Work out the finished part from the listing and answer in its coordinate system (mm). A direction names the side the tool comes from. Round coordinates to 2 decimals unless told otherwise and drop trailing zeros. Write each loop counter-clockwise with the first axis right and the second up, starting at its lowest first coordinate (ties: lowest second). Pieces come first, ordered by that corner, then holes. Notation, with made-up numbers: (-14, -10) - (2, -10) arc R17 cw to (2, -6) - close; hole circle Ø8 at (4.25, 8.5). An arc over 180 degrees is marked (long way). Answer as a JSON object with one key per item and string values.
```python
from build123d import *

# Parameters (mm, degrees)
SKETCH1_R                = 61.7
SEAT_DISC_DEPTH          = 2.8
REAR_STOP_ARC_DEPTH      = 3
SKETCH3_W                = 14
SKETCH3_H                = 23
FRONT_DRAIN_GROOVE_DEPTH = 0.85
SKETCH4_R                = 1
PIN_HOLES_DEPTH          = 1.25


with BuildPart() as part:
    # Sketch1 → Seat_disc (new body)
    with BuildSketch(Plane.XY.offset(72)):
        with Locations((70, 0)):
            Circle(SKETCH1_R)
    extrude(amount=SEAT_DISC_DEPTH)

    # Sketch2 → Rear_stop_arc (add)
    with BuildSketch(Plane.XY.offset(74.8)):
        with BuildLine():
            Line((126.265179381, 15.076209377), (129.597623482, 15.969135083))
            ThreePointArc((129.597623482, 15.969135083), (70, 61.7), (10.402376518, 15.969135083))
            Line((10.402376518, 15.969135083), (13.734820619, 15.076209377))
            ThreePointArc((13.734820619, 15.076209377), (70, 58.25), (126.265179381, 15.076209377))
        make_face()
    extrude(amount=REAR_STOP_ARC_DEPTH)

    # Sketch3 → Front_drain_groove (cut, symmetric)
    with BuildSketch(Plane.XY.offset(74.45)):
        with Locations((70, -51.5)):
            Rectangle(SKETCH3_W, SKETCH3_H)
    extrude(amount=FRONT_DRAIN_GROOVE_DEPTH, both=True, mode=Mode.SUBTRACT)

    # Sketch4 → Pin_holes (cut, symmetric)
    with BuildSketch(Plane.XY.offset(72.75)):
        with Locations((70, 50)):
            Circle(SKETCH4_R)
        with Locations((26.698729811, -25)):
            Circle(SKETCH4_R)
        with Locations((113.301270189, -25)):
            Circle(SKETCH4_R)
    extrude(amount=PIN_HOLES_DEPTH, both=True, mode=Mode.SUBTRACT)


solid = part.part
```
Item 1: Determine the mould class of faces 4 (the flat face through (127.908, 15.516, 76.279)), 5 (the flat face through (70, -51, 73.6)), 6 (the cylindrical face through (61.968, 61.175, 74.215)) for opening direction X: pulls with the +X half, pulls with the -X half, needs draft (parallel to the pull), parting line crosses it, or undercut.
Results found:
{"face 4": "pulls with the +X half", "face 5": "undercut", "face 6": "parting line crosses it"}
Item 2: Each of these flat-tipped pins is pushed along its axis until it touches: P1, Ø2.5, axis at x = 113.3, y = -25, coming from the +Z side; P2, Ø1.3, axis at y = -54.5, z = 74.5, coming from the +X side; P3, Ø0.6, axis at x = 27, y = -25, coming from the -Z side. Where does it stop, or does it pass through?
Results found:
{"P1": "z = 74.8", "P2": "x = 100.12", "P3": "z = 74"}
Item 3: A cutting plane is placed at B-B (x = 23). Write down the section's boundary in (y, z), and give its area (3 significant figures).
Results found:
{"outline": "(-39.97, 72) - (39.97, 72) - (39.97, 77.8) - (34.41, 77.8) - (34.41, 74.8) - (-39.97, 74.8) - close", "area": "241 mm²"}
Item 4: For faces 1 (the cylindrical face through (68.93, 58.24, 76.28)), 2 (the flat face through (70, 59, 77.8)), 3 (the flat face through (12.045, 15.529, 76.279)), determine the directions among +Z, -Z, +X, -X, +Y, -Y from which every point of the face is accessible in a straight line to the end or side of a thin tool.
Results found:
{"face 1": "+Z, -Y", "face 2": "+Z, +X, -X, +Y, -Y", "face 3": "+Z, -X, -Y"}
Item 5: A cutting plane is placed at C-C (y = 31). Write down the section's boundary in (x, z), and give its area (3 significant figures).
Results found:
{"outline": "(16.65, 72) - (123.35, 72) - (123.35, 77.8) - (119.32, 77.8) - (119.32, 74.8) - (20.68, 74.8) - (20.68, 77.8) - (16.65, 77.8) - close", "area": "323 mm²"}
Item 6: A cutting plane is placed at A-A (y = 0). Write down the section's boundary in (x, z).
Results found:
{"outline": "(8.3, 72) - (131.7, 72) - (131.7, 74.8) - (8.3, 74.8) - close"}
Item 7: Consider line 1 along Y through (x, z) = (70, 72.25); line 2 along X through (y, z) = (-53, 73.7); line 3 along Y through (x, z) = (26, 72.85). Determine where each line is inside the solid, lowest interval first.
Results found:
{"line 1": "-61.7 to 49, 51 to 61.7", "line 2": "38.41 to 63, 77 to 101.59", "line 3": "-43.25 to -25.72, -24.28 to 43.25"}
Item 8: A cutting plane is placed at D-D (x = 57.5). Write down the section's boundary in (y, z), and give its area (3 significant figures).
Results found:
{"outline": "(-60.42, 72) - (60.42, 72) - (60.42, 77.8) - (56.89, 77.8) - (56.89, 74.8) - (-60.42, 74.8) - close", "area": "349 mm²"}
